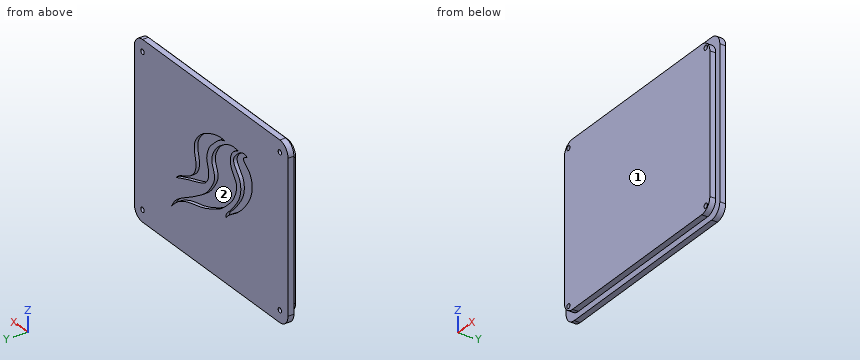
from build123d import *

# Parameters (mm, degrees)
ESBO_O1_W                  = 188
ESBO_O1_H                  = 148
RESSALTO_EXTRUS_O1_DEPTH   = 5
ESBO_O2_W                  = 178
ESBO_O2_H                  = 138
RESSALTO_EXTRUS_O2_DEPTH   = 5
CORTE_EXTRUS_O1_DEPTH      = 3
CORTE_EXTRUS_O2_DEPTH      = 3
CORTE_EXTRUS_O3_START      = 5.999999
CORTE_EXTRUS_O3_DEPTH      = 3.000001
FURO_DE_DI_METRO_4_0_4_1_D = 4
CHANFRO1_SIZE              = 0.025
FILETE1_R                  = 10


with BuildPart() as part:
    # Esboço1 → Ressalto-extrusão1 (new body)
    with BuildSketch(Plane.XZ.offset(5)):
        with Locations((94, -74)):
            Rectangle(ESBO_O1_W, ESBO_O1_H)
    extrude(amount=-RESSALTO_EXTRUS_O1_DEPTH)

    # Esboço2 → Ressalto-extrusão2 (add)
    with BuildSketch(Plane.XZ.offset(5)):
        with Locations((94, -74)):
            Rectangle(ESBO_O2_W, ESBO_O2_H)
    extrude(amount=RESSALTO_EXTRUS_O2_DEPTH)

    # Esboço3 → Corte-extrusão1 (cut)
    with BuildSketch(Plane(origin=(0, 0, 0), x_dir=(-1, 0, 0), z_dir=(0, 1, 0))):
        with BuildLine():
            add(Edge.make_bspline(
                [(-75.851271047, -94.905977801), (-72.853529778, -90.461908235), (-63.518965975, -86.573475907), (-53.388238374, -76.062354108), (-46.202294461, -66.650840181), (-42.933896498, -55.687444915), (-44.842557243, -47.101668287), (-50.660608799, -40.290662898), (-58.64177807, -36.769977477), (-49.631630274, -33.576775134)],
                knots=[0, 0, 0, 0, 0.22173064, 0.36107088, 0.538533699, 0.656521569, 0.776881579, 0.841136845, 1, 1, 1, 1], degree=3))
            add(Edge.make_bspline(
                [(-49.631630274, -33.576775134), (-55.193208686, -30.863794332), (-61.383930126, -35.182265377), (-67.85694371, -43.262736471), (-64.028195245, -49.870932971), (-58.196053752, -55.563823422), (-57.030485514, -66.133339409), (-61.210041506, -75.49236965), (-66.547457609, -81.863728313), (-71.776148718, -88.295991451), (-76.196365931, -90.955926743), (-75.851271047, -94.905977801)],
                knots=[0, 0, 0, 0, 0.190021042, 0.273179635, 0.335508524, 0.444529759, 0.578502017, 0.692991247, 0.817663949, 0.885290163, 1, 1, 1, 1], degree=3))
        make_face()
    extrude(amount=-CORTE_EXTRUS_O1_DEPTH, mode=Mode.SUBTRACT)

    # Esboço4 → Corte-extrusão2 (cut)
    with BuildSketch(Plane(origin=(0, 0, 0), x_dir=(-1, 0, 0), z_dir=(0, 1, 0))):
        with BuildLine():
            add(Edge.make_bspline(
                [(-136.729671692, -91.732742251), (-130.54797809, -89.41900582), (-121.995778776, -86.285522027), (-111.41766579, -83.310038148), (-105.490059757, -81.315624718), (-100.209565482, -78.910124849), (-97.166418624, -73.823248608), (-96.830332763, -68.894438878), (-97.755261853, -63.942155002), (-99.978332244, -59.259888431), (-98.67939373, -53.240415216), (-96.439595754, -47.170244468), (-88.797320177, -40.170304439), (-83.294970154, -34.443536621), (-77.209296676, -33.576775134)],
                knots=[0, 0, 0, 0, 0.208186758, 0.287593338, 0.34598667, 0.40677389, 0.465273363, 0.522640342, 0.558971213, 0.624214432, 0.679618529, 0.747020385, 0.825667459, 1, 1, 1, 1], degree=3))
            add(Edge.make_bspline(
                [(-77.209296676, -33.576775134), (-82.585116536, -32.31898283), (-91.352658464, -34.428249196), (-101.398867055, -38.531561412), (-107.530164378, -43.072555909), (-111.352655789, -47.200724364), (-114.247792048, -51.923301271), (-114.938348234, -56.800502578), (-114.151500445, -61.41688971), (-112.866253897, -65.597847037), (-112.417371236, -70.210515308), (-113.007237755, -74.7648398), (-115.889578157, -79.468708801), (-123.694808489, -85.699371169), (-132.443581982, -86.909139375), (-136.729671692, -91.732742251)],
                knots=[0, 0, 0, 0, 0.166386519, 0.27706617, 0.336739741, 0.403034311, 0.451940723, 0.507330924, 0.55214553, 0.597486466, 0.643567118, 0.69622128, 0.737301428, 0.812802954, 1, 1, 1, 1], degree=3))
        make_face()
    extrude(amount=-CORTE_EXTRUS_O2_DEPTH, mode=Mode.SUBTRACT)

    # Esboço5 → Corte-extrusão3 (cut)
    with BuildSketch(Plane(origin=(0, -8.999999416, 0), x_dir=(1, 0, 0), z_dir=(0, 1, 0)).offset(CORTE_EXTRUS_O3_START)):
        with BuildLine():
            add(Edge.make_bspline(
                [(142.797722166, 118.318760004), (141.55737102, 116.103559652), (139.132967552, 111.773705613), (133.282849534, 107.12676109), (127.016660755, 103.503815432), (120.55072949, 100.15218557), (114.310505573, 96.394806529), (108.124307846, 92.559675632), (102.074067108, 88.493554986), (96.782850849, 83.359171175), (92.821862337, 77.326939474), (88.983167693, 70.724875086), (90.844934858, 63.393230233), (94.274180002, 56.764300619), (91.430089418, 49.523425312), (87.454006301, 43.492143706), (81.590473794, 38.993211516), (75.491955375, 35.081795496), (68.398146179, 32.600302514), (63.514772267, 33.250351232), (61.06257149, 33.576775134)],
                knots=[0, 0, 0, 0, 0.057636738, 0.112657377, 0.168143283, 0.223818375, 0.279375213, 0.335006206, 0.390601607, 0.446300447, 0.501841326, 0.557866933, 0.6118473, 0.666809528, 0.721725073, 0.777322344, 0.83294114, 0.888513668, 0.944016806, 1, 1, 1, 1], degree=3))
            add(Edge.make_bspline(
                [(61.06257149, 33.576775134), (63.70678031, 34.93587517), (68.92788595, 37.619477465), (71.570599658, 46.865300373), (67.920103528, 54.817354375), (61.572954516, 61.557692954), (64.081590616, 70.781691203), (68.213684572, 78.263821244), (74.480339952, 84.318584584), (80.786490273, 90.235655158), (88.573237157, 94.088447273), (96.325623659, 97.780889538), (104.403628291, 100.866438131), (112.828877079, 102.690441809), (121.3012891, 104.295268028), (129.403001338, 107.285492464), (136.990487774, 111.722084003), (140.847014635, 116.10287122), (142.797722166, 118.318760004)],
                knots=[0, 0, 0, 0, 0.062548912, 0.123505555, 0.186160536, 0.247751486, 0.31095589, 0.373508024, 0.436067339, 0.498650764, 0.561041918, 0.62364606, 0.686120194, 0.748656144, 0.811154446, 0.873631853, 0.936080493, 1, 1, 1, 1], degree=3))
        make_face()
    extrude(amount=CORTE_EXTRUS_O3_DEPTH, mode=Mode.SUBTRACT)

    # Furo de diâmetro Ø4.0 (4)1 (through all)
    with Locations(Plane(origin=(0, 0, 0), x_dir=(1, 0, 0), z_dir=(0, 1, 0))):
        with Locations((178, 138), (178, 10), (10, 10), (10, 138)):
            Hole(FURO_DE_DI_METRO_4_0_4_1_D / 2)

    # Chanfro1
    chanfro1_edges = [part.edges().sort_by_distance(p)[0] for p in [
        (12, 0, -138),
        (12, 0, -10),
        (180, 0, -10),
        (180, 0, -138),
    ]]
    chamfer(chanfro1_edges, length=CHANFRO1_SIZE)

    # Filete1
    filete1_edges = [part.edges().sort_by_distance(p)[0] for p in [
        (5, -7.5, -5),
        (5, -7.5, -143),
        (183, -7.5, -143),
        (183, -7.5, -5),
        (0, -2.5, 0),
        (188, -2.5, 0),
        (188, -2.5, -148),
        (0, -2.5, -148),
    ]]
    fillet(filete1_edges, radius=FILETE1_R)


solid = part.part
Geometry check sheet. Reference: the model listing, model coordinates, mm. Face numbers are marked on the shaded views. Coordinates: 2 decimals unless noted, no trailing zeros. Loops run counter-clockwise (first coordinate to the right, second up) from the corner with the lowest first, then second, coordinate; pieces in that order, holes last. Notation, with made-up numbers: (-1.5, -24.5) - (2.5, -24.5) arc R16 ccw to (2.5, -12.5) - close; hole circle Ø7 at (-37, 75.5). An arc over 180 degrees is marked (long way). Use one line per item in the form item = value. Start each with the question number.
Item 1: Thickness scan on probe 1 along Z at (x, y) = (178, -2.75); probe 2 along X at (y, z) = (-4.25, -138); probe 3 along Z at (x, y) = (111.5, -0.5). Record the ranges inside material, lowest first.
Item 2: Mould release check, pull along Z, two halves, no side actions. Record for the marked faces 1 and 2: +Z half, -Z half, draft (parallel to the pull), parting line (faces both ways), or undercut.
Item 3: Section check A-A, the plane x = 154. Enter the section's corners in (y, z), and give its area (3 significant figures).
Item 4: Gauge pin test, flat ends, axial feed: pin 1 (2.5 mm diameter, centred on x = 87.5, y = -8, fed in from +Z); pin 2 (16 mm diameter, centred on x = 59.5, z = -79, fed in from +Y); pin 3 (4 mm diameter, centred on y = -8, z = -65.5, fed in from -X); pin 4 (4 mm diameter, centred on x = 92, y = -7.5, fed in from -Z). Record the tip position at first contact, or that the pin passes through.
Item 5: Section check B-B, the plane y = -7.5. Enter the section's corners in (x, z).
Computed:
q1.probe_1 = -148 to -140, -136 to -12, -8 to 0
q1.probe_2 = 0 to 8, 12 to 176, 180 to 188
q1.probe_3 = -148 to -102.38, -94.64 to -83.28, -47.7 to 0
q2.face_1 = draft
q2.face_2 = undercut
q3.outline = (-10, -143) - (-5, -143) - (-5, -148) - (0, -148) - (0, 0) - (-5, 0) - (-5, -5) - (-10, -5) - close
q3.area = 1,430 mm2
q4.pin_1 = -5
q4.pin_2 = 0
q4.pin_3 = 5
q4.pin_4 = -143
q5.outline = (5, -133) arc R10 ccw to (15, -143) - (173, -143) arc R10 ccw to (183, -133) - (183, -15) arc R10 ccw to (173, -5) - (15, -5) arc R10 ccw to (5, -15) - close; hole circle Ø4 at (10, -138); hole circle Ø4 at (10, -10); hole circle Ø4 at (178, -138); hole circle Ø4 at (178, -10)
